The model under review builds one solid part; all positions refer to its coordinate system, in mm. A direction names the side the tool comes from. Give positions to 0.01 mm unless a question says otherwise; leave off trailing zeros. Write each loop counter-clockwise with the first axis right and the second up, starting at its lowest first coordinate (ties: lowest second). Pieces come first, ordered by that corner, then holes. Notation, with made-up numbers: (52, 15) - (85, 15) arc R27 cw to (85, 40) - close; hole circle Ø3 at (12, 53). An arc over 180 degrees is marked (long way). One line per question, with ' | ' between items. Start each with the question number.
```python
from build123d import *

# Parameters (mm, degrees)
SKETCH_1_R          = 1.45
EXTRUDE_1_DEPTH     = 2
FILLET_1_R          = 3
SKETCH_2_W          = 95
SKETCH_2_H          = 88
SKETCH_2_W_2        = 30
SKETCH_2_H_2        = 101.5
SKETCH_2_W_3        = 87.612976321
SKETCH_2_H_3        = 22.5
SKETCH_2_W_4        = 22
SKETCH_2_H_4        = 51
SKETCH_2_W_5        = 33.612976321
SKETCH_2_H_5        = 20.475952642
CUT_EXTRUDE_1_DEPTH = 10
EXTRUDE_2_DEPTH     = 2
FILLET_2_R          = 4
FILLET_3_R          = 6


with BuildPart() as part:
    # 草图1 → 凸台-拉伸1 (new body)
    with BuildSketch(Plane.XY):
        Polygon((-7.5, 50), (0, 50), (8, 50), (30, 12), (30, 0), (30, -7.5), (90, -7.5), (90, 120.25), (138.75, 120.25), (138.75, 198.75), (8, 198.75), (8, 160), (-8, 160), (-8, 194), (-121, 194), (-121, 82), (-7.5, 82), align=None)
        with Locations((0, 72.5)):
            Circle(SKETCH_1_R, mode=Mode.SUBTRACT)
        with Locations((0, 92.5)):
            Circle(SKETCH_1_R, mode=Mode.SUBTRACT)
        with Locations((0, 152.5)):
            Circle(SKETCH_1_R, mode=Mode.SUBTRACT)
        with Locations((40, 0)):
            Circle(SKETCH_1_R, mode=Mode.SUBTRACT)
        with Locations((80, 0)):
            Circle(SKETCH_1_R, mode=Mode.SUBTRACT)
        with Locations((0, 132.5)):
            Circle(SKETCH_1_R, mode=Mode.SUBTRACT)
        with Locations((-116, 188)):
            Circle(SKETCH_1_R, mode=Mode.SUBTRACT)
        with Locations((-74, 188)):
            Circle(SKETCH_1_R, mode=Mode.SUBTRACT)
        with Locations((-116, 88)):
            Circle(SKETCH_1_R, mode=Mode.SUBTRACT)
        with Locations((-74, 88)):
            Circle(SKETCH_1_R, mode=Mode.SUBTRACT)
        with Locations((-61, 88)):
            Circle(SKETCH_1_R, mode=Mode.SUBTRACT)
        with Locations((-19, 88)):
            Circle(SKETCH_1_R, mode=Mode.SUBTRACT)
        with Locations((-19, 188)):
            Circle(SKETCH_1_R, mode=Mode.SUBTRACT)
        with Locations((-61, 188)):
            Circle(SKETCH_1_R, mode=Mode.SUBTRACT)
        with Locations((14.387023679, 176.862976321)):
            Circle(SKETCH_1_R, mode=Mode.SUBTRACT)
        with Locations((46.862976321, 195.612976321)):
            Circle(SKETCH_1_R, mode=Mode.SUBTRACT)
        with Locations((65.612976321, 163.137023679)):
            Circle(SKETCH_1_R, mode=Mode.SUBTRACT)
        with Locations((33.137023679, 144.387023679)):
            Circle(SKETCH_1_R, mode=Mode.SUBTRACT)
        with Locations((93.25, 163.75)):
            Circle(SKETCH_1_R, mode=Mode.SUBTRACT)
        with Locations((130.75, 163.75)):
            Circle(SKETCH_1_R, mode=Mode.SUBTRACT)
        with Locations((130.75, 126.25)):
            Circle(SKETCH_1_R, mode=Mode.SUBTRACT)
        with Locations((93.25, 126.25)):
            Circle(SKETCH_1_R, mode=Mode.SUBTRACT)
        with BuildLine():
            Line((36, 30), (36, 55))
            ThreePointArc((36, 55), (40, 59), (44, 55))
            Line((44, 55), (44, 30))
            ThreePointArc((44, 30), (40, 26), (36, 30))
        make_face(mode=Mode.SUBTRACT)
        with BuildLine():
            Line((36, 75), (36, 100))
            ThreePointArc((36, 100), (40, 104), (44, 100))
            Line((44, 100), (44, 75))
            ThreePointArc((44, 75), (40, 71), (36, 75))
        make_face(mode=Mode.SUBTRACT)
        with BuildLine():
            Line((10, 123), (20, 123))
            ThreePointArc((20, 123), (23, 120), (20, 117))
            Line((20, 117), (10, 117))
            ThreePointArc((10, 117), (7, 120), (10, 123))
        make_face(mode=Mode.SUBTRACT)
        with BuildLine():
            Line((60, 123), (70, 123))
            ThreePointArc((70, 123), (73, 120), (70, 117))
            Line((70, 117), (60, 117))
            ThreePointArc((60, 117), (57, 120), (60, 123))
        make_face(mode=Mode.SUBTRACT)
    extrude(amount=EXTRUDE_1_DEPTH)

    # 圆角1
    fillet_1_edges = [part.edges().sort_by_distance(p)[0] for p in [
        (-7.5, 82, 1),
        (-121, 82, 1),
        (-121, 194, 1),
        (-8, 194, 1),
        (-8, 160, 1),
        (8, 160, 1),
        (8, 198.75, 1),
        (138.75, 198.75, 1),
        (138.75, 120.25, 1),
        (90, 120.25, 1),
        (90, -7.5, 1),
        (30, -7.5, 1),
        (30, 12, 1),
        (8, 50, 1),
        (-7.5, 50, 1),
    ]]
    fillet(fillet_1_edges, radius=FILLET_1_R)

    # 草图2 → 切除-拉伸1 (cut)
    with BuildSketch(Plane.XY.offset(2)):
        with Locations((-67.5, 138)):
            Rectangle(SKETCH_2_W, SKETCH_2_H)
        Polygon((58.75, 198.75), (74.338457268, 171.75), (138.75, 171.75), (138.75, 198.75), align=None)
        with Locations((67, 58.25)):
            Rectangle(SKETCH_2_W_2, SKETCH_2_H_2)
        with Locations((88.94351184, 146.5)):
            Rectangle(SKETCH_2_W_3, SKETCH_2_H_3)
        with Locations((17, 83.5)):
            Rectangle(SKETCH_2_W_4, SKETCH_2_H_4)
        with Locations((36.806488161, 177.375)):
            Rectangle(SKETCH_2_W_5, SKETCH_2_H_5)
    extrude(amount=-CUT_EXTRUDE_1_DEPTH, mode=Mode.SUBTRACT)

    # 草图3 → 凸台-拉伸2 (add)
    with BuildSketch(Plane.XY):
        Polygon((82, 109), (56.127900679, 7.5), (52, 7.5), (77.872099321, 109), align=None)
        Polygon((-20, 94), (-115, 175.415073416), (-115, 182), (-20, 100.584926584), align=None)
    extrude(amount=EXTRUDE_2_DEPTH)

    # 圆角2
    fillet_2_edges = [part.edges().sort_by_distance(p)[0] for p in [
        (-20, 182, 1),
        (-20, 94, 1),
        (-115, 94, 1),
        (-115, 182, 1),
        (53.612976321, 187.612976321, 1),
        (53.612976321, 167.137023679, 1),
        (20, 167.137023679, 1),
        (20, 187.612976321, 1),
        (82, 109, 1),
        (82, 7.5, 1),
        (52, 7.5, 1),
        (52, 109, 1),
        (132.75, 157.75, 1),
        (132.75, 135.25, 1),
        (45.137023679, 135.25, 1),
        (45.137023679, 157.75, 1),
        (28, 109, 1),
        (28, 58, 1),
        (6, 58, 1),
        (6, 109, 1),
        (77.872099321, 109, 1),
        (56.127900679, 7.5, 1),
        (-20, 100.584926584, 1),
        (-115, 175.415073416, 1),
    ]]
    fillet(fillet_2_edges, radius=FILLET_2_R)

    # 圆角3
    fillet_3_edges = [part.edges().sort_by_distance(p)[0] for p in [
        (138.75, 171.75, 1),
        (74.338457268, 171.75, 1),
        (58.75, 198.75, 1),
    ]]
    fillet(fillet_3_edges, radius=FILLET_3_R)


solid = part.part
```
Item 1: Machinability: for faces 5 (the flat face through (66.459, 185.397, 1.014)), 6 (the flat face through (-67.257, 141.084, 0.986)), which of the approach directions +Z, -Z, +X, -X, +Y, -Y give a long, thin tool a straight path to every point of the face, cutting with its end or side? Answer none if there is none.
Item 2: The part is to be moulded in two halves that separate along Y. For faces 1 (the flat face through (19, 31, 1)), 2 (the flat face through (19, 111, 2)), 3 (the cylindrical face through (136.946, 170.039, 0.986)), 4 (the flat face through (68.121, 70.746, 0.986)), say which applies: +Y half, -Y half, draft (parallel to the pull), parting line (faces both ways), or undercut.
Item 3: Clearance check with flat-ended pins moving along their axes: P1, Ø4, axis at x = 93.25, y = 126.25, coming from the +Z side; P2, Ø1, axis at x = -10, z = 1, coming from the -Y side; P3, Ø1, axis at y = 37, z = 1, coming from the +X side; P4, Ø1, axis at x = 63.5, z = 0.5, coming from the +Y side. State where each tip first meets the part, or that it passes through.
Item 4: For probe 1 along Y at (x, z) = (40, 1.5); probe 2 along Y at (x, z) = (33.5, 1.5); probe 3 along Y at (x, z) = (0, 0.6), list the stretches that pass through material, from the lowest coordinate up.
Item 5: Take a section at A-A (x = 112.5). Give the boundary of the cut face in (y, z).
Item 6: Take a section at B-B (y = 42.5). Give the boundary of the cut face in (x, z).
Item 7: Take a section at C-C (z = 0.5). State how many separate pieces and enclosed holes the cut face has, plus the area to 3 significant figures.
Check sheet entries:
1) face 5: +Z, -Z, +X, +Y | face 6: +Z, -Z
2) face 1: -Y half | face 2: draft | face 3: +Y half | face 4: undercut
3) P1: stops at z = 2 | P2: stops at y = 81.83 | P3: stops at x = 90 | P4: stops at y = 191.39
4) probe 1: y = -7.5 to -1.45, 1.45 to 26, 59 to 71, 104 to 167.14, 187.61 to 198.75 | probe 2: y = -7.5 to 142.98, 145.79 to 167.14, 187.61 to 198.75 | probe 3: y = 50 to 71.05, 73.95 to 91.05, 93.95 to 131.05, 133.95 to 151.05, 153.95 to 160
5) outline: (120.25, 0) - (135.25, 0) - (135.25, 2) - (120.25, 2) - close; (157.75, 0) - (171.75, 0) - (171.75, 2) - (157.75, 2) - close
6) outline: (12.34, 0) - (36, 0) - (36, 2) - (12.34, 2) - close; (44, 0) - (52, 0) - (52, 2) - (44, 2) - close; (60.92, 0) - (65.05, 0) - (65.05, 2) - (60.92, 2) - close; (82, 0) - (90, 0) - (90, 2) - (82, 2) - close
7) separate pieces: 1 | enclosed holes: 33 | area: 17,700 mm^2
